For this review, take the finished solid that the model builds, in its own axes (mm). Face numbers are marked on the shaded views. A direction names the side the tool comes from. Round coordinates to 2 decimals unless told otherwise and drop trailing zeros. Order: outer loops, then holes, each group sorted by start corner. A loop starts at its lowest first (then second) coordinate and runs counter-clockwise, first axis right, second up. Notation, with made-up numbers: M 25.5,14.5 L 76.5,14.5 A26 cw 76.5,51.5 Z; hole C 80.5,44 d11. An arc over 180 degrees is marked long. Put each result on its own line as item: value.
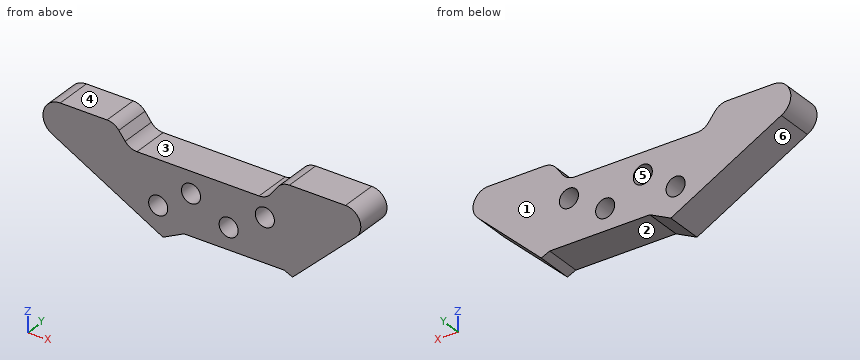
from build123d import *

# Parameters (mm, degrees)
SKETCH1_R           = 3.2639
BOSS_EXTRUDE1_DEPTH = 12.7


with BuildPart() as part:
    # Sketch1 → Boss-Extrude1 (new body)
    with BuildSketch(Plane(origin=(0, 0, 0), x_dir=(1, 0, 0), z_dir=(0, 1, 0))):
        with BuildLine():
            Line((98.733031573, -68.985835228), (100.942599672, -71.978006872))
            ThreePointArc((100.942599672, -71.978006872), (102.740427245, -73.495514847), (105.029143887, -74.040299732))
            Line((105.029143887, -74.040299732), (124.201892168, -74.040299732))
            ThreePointArc((124.201892168, -74.040299732), (129.062693158, -70.745465469), (127.802444272, -65.010041176))
            Line((127.802444272, -65.010041176), (106.094318665, -44.426787292))
            Line((106.094318665, -44.426787292), (103.19820861, -45.713487798))
            Line((103.19820861, -45.713487798), (68.977352979, -45.713487798))
            Line((68.977352979, -45.713487798), (61.792374607, -42.131557151))
            Line((61.792374607, -42.131557151), (24.038270246, -62.563232545))
            ThreePointArc((24.038270246, -62.563232545), (20.915380805, -69.188017292), (26.654079797, -73.738571684))
            Line((26.654079797, -73.738571684), (42.658611745, -73.738571684))
            ThreePointArc((42.658611745, -73.738571684), (44.904764604, -73.215017375), (46.687932027, -71.752271422))
            Line((46.687932027, -71.752271422), (48.870340124, -68.909842629))
            ThreePointArc((48.870340124, -68.909842629), (50.653507547, -67.447096676), (52.899660406, -66.923542367))
            Line((52.899660406, -66.923542367), (94.646487358, -66.923542367))
            ThreePointArc((94.646487358, -66.923542367), (96.935204, -67.468327252), (98.733031573, -68.985835228))
        make_face()
        with Locations((60.150170667, -51.891201826)):
            Circle(SKETCH1_R, mode=Mode.SUBTRACT)
        with Locations((71.3764156, -59.641849895)):
            Circle(SKETCH1_R, mode=Mode.SUBTRACT)
        with Locations((84.237729699, -53.077081169)):
            Circle(SKETCH1_R, mode=Mode.SUBTRACT)
        with Locations((96.63028976, -60.633621731)):
            Circle(SKETCH1_R, mode=Mode.SUBTRACT)
    extrude(amount=BOSS_EXTRUDE1_DEPTH)


solid = part.part
(1) Add section C-C on x = 84.5. Give the boundary of the cut face in (y, z), then the cut area to 3 significant figures.
A:
outline: M 0,45.71 L 12.7,45.71 L 12.7,49.82 L 0,49.82 Z; M 0,56.33 L 12.7,56.33 L 12.7,66.92 L 0,66.92 Z
area: 187 mm2
(2) Draft analysis for pull direction X (two halves, no side actions). For the marked faces 4, 5 and 6, state which applies: released by +X, released by -X, zero draft, split by the parting line, or undercut.
A:
face 4: zero draft
face 5: undercut
face 6: released by -X
(3) Add section D-D on x = 117. Give the boundary of the cut face in (y, z).
A:
outline: M 0,54.77 L 12.7,54.77 L 12.7,74.04 L 0,74.04 Z
(4) Add section B-B on y = 11.5. Give the boundary of the cut face in (x, z), then the cut area to 3 significant figures.
A:
outline: M 24.04,62.56 L 61.79,42.13 L 68.98,45.71 L 103.2,45.71 L 106.09,44.43 L 127.8,65.01 A5.23 ccw 124.2,74.04 L 105.03,74.04 A5.08 ccw 100.94,71.98 L 98.73,68.99 A5.08 cw 94.65,66.92 L 52.9,66.92 A5.08 cw 48.87,68.91 L 46.69,71.75 A5.08 ccw 42.66,73.74 L 26.65,73.74 A5.89 ccw Z; hole C 60.15,51.89 d6.53; hole C 71.38,59.64 d6.53; hole C 84.24,53.08 d6.53; hole C 96.63,60.63 d6.53
area: 2,030 mm2
(5) For the marked faces 1, 2 and 3, list the 3-axis set-ups (+Z, -Z, +X, -X, +Y, -Y) from which the entire face can be reached by the end or side of a thin tool; tool diameter is ignored.
A:
face 1: +Z, -Z, +X, -X, +Y
face 2: -Z, +Y, -Y
face 3: +Z, +Y, -Y
(6) To check wall thickness, follow L1, parallel to X at y = 9, z = 58; L2, parallel to X at y = 7.75, z = 51.5; L3, parallel to Z at x = 61, y = 0.5. State the ranges of each line that lie inside material, in increasing order.
A:
L1: x = 32.47 to 68.56, 74.2 to 94.7, 98.56 to 120.41
L2: x = 44.48 to 56.91, 63.39 to 81.38, 87.1 to 113.55
L3: z = 42.56 to 48.74, 55.04 to 66.92
(7) Insertion check: pin 1 Ø6 at (x, z) = (60.15, 51.89) entering from -Y; pin 2 Ø2 at (x, y) = (96, 10) entering from +Z; pin 3 Ø1.5 at (y, z) = (9.5, 60) entering from -X; pin 4 Ø4 at (x, y) = (70, 4) entering from +Z. Each pin has a flat end and moves straight along its axis. Give the tip position at first contact, or say it passes through.
A:
pin 1: passes through
pin 2: stops at z = 67.5
pin 3: stops at x = 27.39
pin 4: stops at z = 66.92
(8) Add section A-A on x = 97.5. Give the boundary of the cut face in (y, z), then the cut area to 3 significant figures.
A:
outline: M 0,45.71 L 12.7,45.71 L 12.7,57.49 L 0,57.49 Z; M 0,63.78 L 12.7,63.78 L 12.7,67.8 L 0,67.8 Z
area: 201 mm2
